Work out the finished part from the listing and answer in its coordinate system (mm). Face numbers are marked on the shaded views. A direction names the side the tool comes from. Give positions to 0.01 mm unless a question says otherwise; leave off trailing zeros. Loops run counter-clockwise (first coordinate to the right, second up) from the corner with the lowest first, then second, coordinate; pieces in that order, holes last.
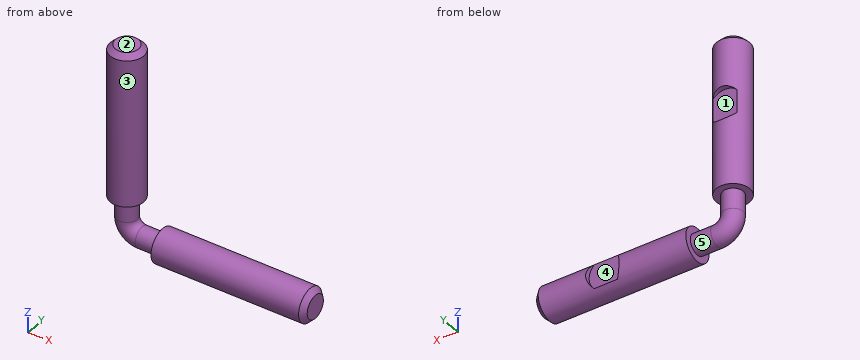
Autodesk Inventor part; units mm, degrees
ref_plane "Work Plane1" through (0, 0, 7) normal (0, 0, 1) x (1, 0, 0)
ref_plane "Work Plane2" through (0, 3.285, 7) normal (0, 1, 0) x (-1, 0, 0)
ref_plane "YZ Plane" through (0, 0, 0) normal (1, 0, 0) x (0, 1, 0)
ref_plane "Work Plane1" through (0, 0, 7) normal (0, 0, 1) x (1, 0, 0)
sketch "Sketch1" plane through (0, 0, 7) normal (0, 0, 1) x (1, 0, 0)
  circle A0 centre (0, 0) radius 3.285
  dimension "d0" = 6.57
extrude "Extrusion1" add sketch "Sketch1" along normal blind 30
chamfer "Chamfer1" distance 1 angle 45 1 edges at (-3.285, 0, 37)
ref_plane "Work Plane2" through (0, 3.285, 7) normal (0, 1, 0) x (-1, 0, 0)
sketch "Sketch2" plane through (0, 3.285, 7) normal (0, 1, 0) x (-1, 0, 0)
  line L0 (3.285, 0) -> (3.285, 29)
  line L1 (-3.285, 0) -> (-3.285, 29)
  circle A0 centre (0, 16.4) radius 3.285
  point P0 (0, -7)
  dimension "d10" = 23.4
extrude "Extrusion2" cut sketch "Sketch2" against normal blind 1
pattern_circular "Circular Pattern1" count 2 over 90 about axis through (0, -10, 0) along (0, 1, 0) of "Extrusion1", "Chamfer1", "Extrusion2"
sketch "Sketch3" plane through (0, 0, 0) normal (0, 1, 0) x (-1, 0, 0)
  line L0 (-7, -3.285) -> (-7, 3.285)
  line L1 (-3.285, 7) -> (3.285, 7)
  line L2 (-7, 0) -> (-3, 0)
  line L3 (0, 3) -> (0, 7)
  arc A0 (-3, 0) -> (0, 3) centre (-3, 3) ccw
  dimension "d13" = 3
sketch "Sketch4" plane through (0, 0, 7) normal (0, 0, -1) x (-1, 0, 0)
  circle A0 centre (0, 0) radius 3.285 construction
  circle A1 centre (0, 0) radius 2
  dimension "d14" = 4
sweep "Sweep1" add profiles "Sketch4" path "Sketch3" path curves L3 A0 L2
equation "\"BendRadius\" = Thickness"
equation "\"BendReliefWidth\" = Thickness"
equation "\"BendReliefDepth\" = 0.5 * Thickness"
equation "\"CornerReliefSize\" = 4 * Thickness"
equation "\"MinimumRemnant\" = 2 * Thickness"
equation "\"TransitionRadius\" = BendRadius"
equation "\"JacobiRadiusSize\" = Thickness"
equation "\"GapSize\" = Thickness"
properties part number "20-128Z1"
Q1. Which of the six approach directions +Z, -Z, +X, -X, +Y, -Y give full straight-line access (tool end or side, diameter ignored) to the marked faces 4 and 5?
Q2. Consider line 1 along Z through (x, y) = (14, -0.25); line 2 along X through (y, z) = (-1, 22.5); line 3 along Z through (x, y) = (-1, -0.75). Determine where each line is inside the solid, lowest interval first.
Q3. Determine the mould class of the marked faces 1, 2 and 3 for opening direction X: +X half, -X half, draft (parallel to the pull), parting line (faces both ways), or undercut.
Q4. Section D-D on z = 25 is taken. Give the vertices of the cut face in (x, y) (3 decimals), plus the area to 3 significant figures.
Q5. Section A-A on y = 0 is taken. Give the vertices of the cut face in (x, z) (3 decimals), plus the area to 3 significant figures.
Q6. Section B-B on z = 12 is taken. Give the vertices of the cut face in (x, y) (3 decimals), plus the area to 3 significant figures.
Q7. Given pin 1 (3 mm diameter, centred on y = -2.5, z = 19.5, fed in from +X); pin 2 (1.4 mm diameter, centred on x = 1, z = 24.5, fed in from +Y) (3 decimals); pin 3 (5 mm diameter, centred on x = 7, z = 3.5, fed in from +Y), each flat-ended and moving along its own axis, determine where each tip first touches the part or whether it passes through.
Check result:
1. face 4: +Y
1. face 5: none
2. line 1: z = -3.28 to 3.28
2. line 2: x = -3.13 to 3.13
2. line 3: z = 0.25 to 37
3. face 1: undercut
3. face 2: draft
3. face 3: parting line
4. outline: (-2.36, 2.285) arc R3.285 ccw (long way) to (2.36, 2.285) - close
4. area: 30.6 mm2
5. outline: (-3.285, 7) - (-2, 7) - (-2, 3) arc R5 ccw to (3, -2) - (7, -2) - (7, -3.285) - (36, -3.285) - (37, -2.285) - (37, 2.285) - (36, 3.285) - (7, 3.285) - (7, 2) - (3, 2) arc R1 cw to (2, 3) - (2, 7) - (3.285, 7) - (3.285, 36) - (2.285, 37) - (-2.285, 37) - (-3.285, 36) - close
5. area: 443 mm2
6. outline: circle Ø6.57 at (0, 0)
6. area: 33.9 mm2
7. pin 1: stops at x = 3.13
7. pin 2: stops at y = 2.285
7. pin 3: stops at y = 3.13
